```python
from build123d import *

# Parameters (mm, degrees)
F1_DEPTH = 63.5
F0_W     = 25.4
F0_H     = 19.05
F2_DEPTH = 25.4
F3_DEPTH = 7.9375
F5_R     = 6.35


with BuildPart() as f1:
    # F0 (on Front) → F1 (new body, symmetric)
    with BuildSketch(Plane.XZ):
        Polygon((41.275, 8.7261183647), (41.275, 9.525), (22.225, 9.525), (-41.275, 9.525), (-41.275, -9.525), (41.275, -9.525), align=None)
    extrude(amount=F1_DEPTH, both=True)

    # F0 (on Front) → F2 (join, symmetric)
    with BuildSketch(Plane.XZ):
        with BuildLine():
            Line((22.225, 9.525), (41.275, 9.525))
            Line((41.275, 9.525), (41.275, 27.0002))
            ThreePointArc((41.275, 27.0002), (45.9246798487, 38.2255201513), (57.15, 42.8752))
            Line((57.15, 42.8752), (60.325, 42.8752))
            Line((60.325, 42.8752), (60.325, 61.9252))
            Line((60.325, 61.9252), (57.15, 61.9252))
            ThreePointArc((57.15, 61.9252), (32.4542956671, 51.6959043329), (22.225, 27.0002))
            Line((22.225, 27.0002), (22.225, 9.525))
        make_face()
        with Locations((73.025, 52.4002)):
            Rectangle(F0_W, F0_H)
    extrude(amount=F2_DEPTH, both=True)

    # F0 (on Front) → F3 (join, symmetric)
    with BuildSketch(Plane.XZ):
        with BuildLine():
            Line((-41.275, 9.525), (22.225, 9.525))
            Line((22.225, 9.525), (22.225, 27.0002))
            ThreePointArc((22.225, 27.0002), (32.4542956671, 51.6959043329), (57.15, 61.9252))
            add(Edge.make_bspline(
                [(-41.275, 9.525), (12.6994326711, 36.1836515367), (13.9212344627, 62.6314580441), (57.15, 61.9252)],
                knots=[0, 0, 0, 0, 111.5045361635, 111.5045361635, 111.5045361635, 111.5045361635], degree=3))
        make_face()
    extrude(amount=F3_DEPTH, both=True)

    # F0 (on Front) → F4 (revolve)
    with BuildSketch(Plane.XZ):
        Polygon((85.725, 61.9252), (85.725, 42.8752), (85.725, 38.1), (111.125, 38.1), (111.125, 66.675), (85.725, 66.675), align=None)
    revolve(axis=Axis((85.725, 0, 52.3875), (0, 0, -1)))

    # F5
    f5_edges = [f1.edges().sort_by_distance(p)[0] for p in [
        (41.275, -63.5, 0),
        (-41.275, -63.5, 0),
        (-41.275, 63.5, 0),
        (41.275, 63.5, 0),
    ]]
    fillet(f5_edges, radius=F5_R)


solid = f1.part
```
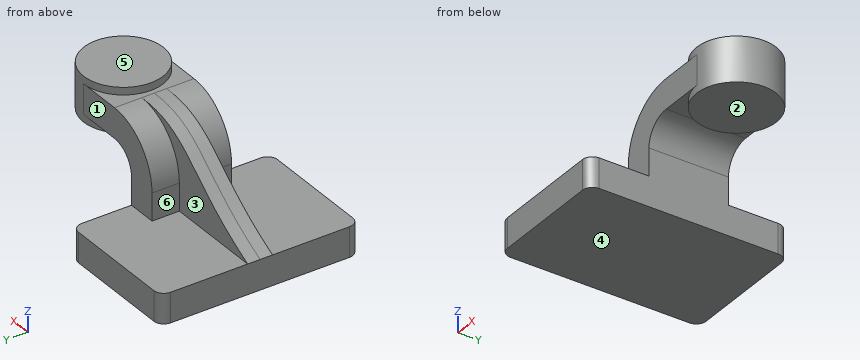
Input: part model. Units: mm. Frame: model coordinates. Face numbers are marked on the shaded views. A direction names the side the tool comes from. Round coordinates to 2 decimals unless told otherwise and drop trailing zeros. Loops run counter-clockwise (first coordinate to the right, second up) from the corner with the lowest first, then second, coordinate; pieces in that order, holes last. Notation, with made-up numbers: (48.25, 5.25) - (99.25, 5.25) arc R17 ccw to (99.25, 20.25) - close; hole circle Ø9 at (17.5, 73). An arc over 180 degrees is marked (long way). One line per item, written item: value. Start each with the question number.
(1) Section A-A, the plane y = -45. Return loops of the section in (x, z) (3 decimals).
(2) Section B-B, the plane x = 90. Return loops of the section in (y, z) (3 decimals), plus the area to 3 significant figures.
(3) Section C-C, the plane y = -21.5. Return loops of the section in (x, z) (3 decimals), plus the area to 3 significant figures.
(4) Access query for the marked faces 1, 2 and 3. Directions: +Z, -Z, +X, -X, +Y, -Y. A direction counts if a zero-diameter tool reaches every point of the face in a straight line with its end or side. Return the directions, or none.
(5) Contact query for flat-ended pins moving along their axis: P1, Ø11, axis at y = -5, z = 8, coming from the +X side (3 decimals); P2, Ø16.5, axis at x = 6.5, y = 25, coming from the +Z side (3 decimals); P3, Ø5, axis at y = -13, z = 19, coming from the -X side (3 decimals). Output: stop coordinate, or through.
(6) Ray query, line 1 (Z direction, x = 85, y = -4.5) (3 decimals); line 2 (X direction, y = -26, z = -2.5) (3 decimals); line 3 (Z direction, x = 18, y = 20.5) (3 decimals). Return the intervals inside material, ascending. Write a range as [from, to].
(7) Draft query along Z for the marked faces 4, 5 and 6. Return one class per face: +Z half, -Z half, draft (parallel to the pull), parting line (faces both ways), or undercut.
Results below:
1. outline: (-41.275, -9.525) - (41.275, -9.525) - (41.275, 9.525) - (-41.275, 9.525) - close
2. outline: (-25.038, 38.1) - (25.038, 38.1) - (25.038, 66.675) - (-25.038, 66.675) - close
2. area: 1,430 mm^2
3. outline: (-41.275, -9.525) - (41.275, -9.525) - (41.275, 27) arc R15.875 cw to (57.15, 42.875) - (72.201, 42.875) - (72.201, 38.1) - (99.249, 38.1) - (99.249, 66.675) - (72.201, 66.675) - (72.201, 61.925) - (57.15, 61.925) arc R34.925 ccw to (22.225, 27) - (22.225, 9.525) - (-41.275, 9.525) - close
3. area: 3,730 mm^2
4. face 1: +Z, +X, -X, +Y
4. face 2: -Z, +X, +Y, -Y
4. face 3: +Z, -X, +Y
5. P1: x = 41.275
5. P2: z = 9.525
5. P3: x = 22.225
6. line 1: [38.1, 66.675]
6. line 2: [-41.275, 41.275]
6. line 3: [-9.525, 9.525]
7. face 4: -Z half
7. face 5: +Z half
7. face 6: draft
